```python
from build123d import *

# Parameters (mm, degrees)
CYLINDER003_R     = 2.5
CYLINDER003_DEPTH = 11.5
CYLINDER022_R     = 5
CYLINDER022_DEPTH = 11.5
CYLINDER002_R     = 10
CYLINDER002_DEPTH = 4


with BuildPart() as cylinder003:
    # Cylinder003 → Cylinder003 (new body)
    with BuildSketch(Plane.XY):
        Circle(CYLINDER003_R)
    extrude(amount=CYLINDER003_DEPTH)


with BuildPart() as cylinder022:
    # Cylinder022 → Cylinder022 (new body)
    with BuildSketch(Plane.XY):
        Circle(CYLINDER022_R)
    extrude(amount=CYLINDER022_DEPTH)


with BuildPart() as obj1:
    # Cylinder002 → Cylinder002 (new body)
    with BuildSketch(Plane.XY):
        Circle(CYLINDER002_R)
    extrude(amount=CYLINDER002_DEPTH)

    # Fusion001018017021: union Cylinder022
    add(cylinder022.part)

    # Cut: cut Cylinder003
    add(cylinder003.part, mode=Mode.SUBTRACT)


solid = obj1.part
```
For this review, take the finished solid that the model builds, in its own axes (mm). A direction names the side the tool comes from. Give positions to 0.01 mm unless a question says otherwise; leave off trailing zeros. Order: outer loops, then holes, each group sorted by start corner. A loop starts at its lowest first (then second) coordinate and runs counter-clockwise, first axis right, second up.
1) Insertion check: pin 1 (1 mm diameter, centred on x = 4.5, y = 7.5, fed in from +Z); pin 2 (1 mm diameter, centred on x = 6, z = 1.5, fed in from +Y); pin 3 (3 mm diameter, centred on y = -5.5, z = 2, fed in from -X); pin 4 (4.5 mm diameter, centred on x = 0, y = 0, fed in from -Z). Each pin has a flat end and moves straight along its axis. Give the tip position at first contact, or say it passes through.
2) Wall thickness on line 1 (Y direction, x = 0, z = 6); line 2 (Z direction, x = 2.75, y = -4.5); line 3 (X direction, y = 1.25, z = 6): over which ranges is each line inside the solid? List them lowest first.
3) The part is to be moulded in two halves that separate along Y. For faces 1 (the face through (2, -2, 11.5)), 2 (the face through (-1.08, -4.88, 7.7)), 3 (the face through (-0.54, -2.44, 5.67)), say which applies: released by +Y, released by -Y, zero draft, split by the parting line, or undercut.
4) Take a section at D-D (y = -4). Give the boundary of the cut face in (x, z).
5) For faces 4 (the face through (-5, -2, 4)), 5 (the face through (-2.17, -9.76, 1.97)), list the 3-axis set-ups (+Z, -Z, +X, -X, +Y, -Y) from which the entire face can be reached by the end or side of a thin tool; tool diameter is ignored.
6) Take a section at C-C (z = 4.5). Give the boundary of the cut face in (x, y).
7) Take a section at A-A (y = 0). Give the boundary of the cut face in (x, z).
Derived:
1. pin 1: stops at z = 4
1. pin 2: stops at y = 8.35
1. pin 3: stops at x = -9.17
1. pin 4: passes through
2. line 1: y = -5 to -2.5, 2.5 to 5
2. line 2: z = 0 to 4
2. line 3: x = -4.84 to -2.17, 2.17 to 4.84
3. face 1: zero draft
3. face 2: split by the parting line
3. face 3: undercut
4. outline: (-9.17, 0) - (9.17, 0) - (9.17, 4) - (3, 4) - (3, 11.5) - (-3, 11.5) - (-3, 4) - (-9.17, 4) - close
5. face 4: +Z
5. face 5: +Z, -Z
6. outline: circle Ø10 at (0, 0); hole circle Ø5 at (0, 0)
7. outline: (-10, 0) - (-2.5, 0) - (-2.5, 11.5) - (-5, 11.5) - (-5, 4) - (-10, 4) - close; (2.5, 0) - (10, 0) - (10, 4) - (5, 4) - (5, 11.5) - (2.5, 11.5) - close
